```python
from build123d import *

# Parameters (mm, degrees)
F0_W     = 15
F0_H     = 15
F2_DEPTH = 1.2
F3_W     = 1.2
F3_H     = 15
F4_DEPTH = 10
F5_R     = 1
F6_D     = 5.5


with BuildPart() as f2:
    # F0 (on Top) → F2 (new body)
    with BuildSketch(Plane.XY):
        with Locations((-7.5, -26.9438664615)):
            Rectangle(F0_W, F0_H)
    extrude(amount=F2_DEPTH)

    # F3 (on face) → F4 (join)
    with BuildSketch(Plane.XY):
        with Locations((-0.6, -26.9438664615)):
            Rectangle(F3_W, F3_H)
        with Locations((-14.4, -26.9438664615)):
            Rectangle(F3_W, F3_H)
    extrude(amount=-F4_DEPTH)

    # F5
    f5_edges = [f2.edges().sort_by_distance(p)[0] for p in [
        (-15, -26.943866, 1.2),
        (0, -26.943866, 1.2),
        (-1.2, -26.943866, 0),
        (-13.8, -26.943866, 0),
    ]]
    fillet(f5_edges, radius=F5_R)

    # F6 (through all)
    with Locations(Plane(origin=(0, 0, 0), x_dir=(1, 0, 0), z_dir=(0, 0, -1))):
        with Locations((-7.5, 26.9438664615)):
            Hole(F6_D / 2)


solid = f2.part
```
CAD build for the part. Positions are in the model's coordinates, mm. A direction names the side the tool comes from. Coordinates: 2 decimals unless noted, no trailing zeros. Order: outer loops, then holes, each group sorted by start corner. A loop starts at its lowest first (then second) coordinate and runs counter-clockwise, first axis right, second up. Notation, with made-up numbers: (-11, 40.25) - (7, 40.25) arc R7 ccw to (7, 46.25) - close; hole circle Ø6 at (-22.5, -13.5). An arc over 180 degrees is marked (long way). Answer in a Markdown table with one row per item.
1. Slice it at A-A, the plane z = -4.5. List the corners of the cut face in (x, y).
Answer:
| item | result |
|---|---|
| outline | (-15, -34.44) - (-13.8, -34.44) - (-13.8, -19.44) - (-15, -19.44) - close; (-1.2, -34.44) - (0, -34.44) - (0, -19.44) - (-1.2, -19.44) - close |
2. Flat gauge pins, fed straight in: P1, Ø5, axis at x = -7.5, y = -26.94, coming from the +Z side; P2, Ø5.5, axis at x = -9.5, y = -24.5, coming from the -Z side. Where does each tip first touch, or does it go through?
Answer:
| item | result |
|---|---|
| P1 | through |
| P2 | z = 0 |
3. Drill centre lines: L1, parallel to Y at x = -7.5, z = 0.5; L2, parallel to X at y = -27, z = -9.5; L3, parallel to Z at x = -8.5, y = -22.75. Where is each one in solid material? Low to high. Write a range as from..to.
Answer:
| item | result |
|---|---|
| L1 | -34.44..-29.69, -24.19..-19.44 |
| L2 | -15..-13.8, -1.2..0 |
| L3 | 0..1.2 |
4. Slice it at B-B, the plane x = -7.5. List the corners of the cut face in (y, z), then the cut area to 3 significant figures.
Answer:
| item | result |
|---|---|
| outline | (-34.44, 0) - (-29.69, 0) - (-29.69, 1.2) - (-34.44, 1.2) - close; (-24.19, 0) - (-19.44, 0) - (-19.44, 1.2) - (-24.19, 1.2) - close |
| area | 11.4 mm² |
5. Slice it at D-D, the plane y = -32.5. List the corners of the cut face in (x, z), then the cut area to 3 significant figures.
Answer:
| item | result |
|---|---|
| outline | (-15, -10) - (-13.8, -10) - (-13.8, -1) arc R1 cw to (-12.8, 0) - (-2.2, 0) arc R1 cw to (-1.2, -1) - (-1.2, -10) - (0, -10) - (0, 0.2) arc R1 ccw to (-1, 1.2) - (-14, 1.2) arc R1 ccw to (-15, 0.2) - close |
| area | 42.0 mm² |
6. Pull direction X, two halves, no side cores. Call faces 1 (the face through (-10.5, -26.8, 1.2)), 2 (the face through (-0.285, -26.839, 0.899)), 3 (the face through (-13.8, -27, -5)), 4 (the face through (-10, -29, 0)): +X half, -X half, draft (parallel to the pull), parting line (faces both ways), or undercut.
Answer:
| item | result |
|---|---|
| face 1 | draft |
| face 2 | +X half |
| face 3 | undercut |
| face 4 | undercut |
7. Slice it at C-C, the plane y = -26. List the corners of the cut face in (x, z).
Answer:
| item | result |
|---|---|
| outline | (-15, -10) - (-13.8, -10) - (-13.8, -1) arc R1 cw to (-12.8, 0) - (-10.08, 0) - (-10.08, 1.2) - (-14, 1.2) arc R1 ccw to (-15, 0.2) - close; (-4.92, 0) - (-2.2, 0) arc R1 cw to (-1.2, -1) - (-1.2, -10) - (0, -10) - (0, 0.2) arc R1 ccw to (-1, 1.2) - (-4.92, 1.2) - close |
8. 3-axis set-ups, long thin cutter, end or side, ignore diameter. For faces 5 (the face through (-13.515, -26.839, -0.301)), 6 (the face through (-10.04, -25.89, 0.61)): which of +Z, -Z, +X, -X, +Y, -Y reach the whole face in a straight line?
Answer:
| item | result |
|---|---|
| face 5 | -Z, +Y, -Y |
| face 6 | +Z, -Z |
